from build123d import *

# Parameters (mm, degrees)
SKETCH1_W           = 45.974
SKETCH1_H           = 31.496
BOSS_EXTRUDE2_DEPTH = 17.78
BOSS_EXTRUDE6_DEPTH = 3.302


with BuildPart() as part:
    # Sketch1 → Boss-Extrude2 (new body)
    with BuildSketch(Plane(origin=(0, 0, 0), x_dir=(1, 0, 0), z_dir=(0, 1, 0))):
        with Locations((1.215537396, -0.182473566)):
            Rectangle(SKETCH1_W, SKETCH1_H)
    extrude(amount=BOSS_EXTRUDE2_DEPTH)

    # Sketch2 → Boss-Extrude6 (add)
    with BuildSketch(Plane.XZ):
        with BuildLine():
            Line((-21.771462604, 6.913473566), (-21.771462604, -6.548526434))
            Line((-21.771462604, -6.548526434), (-30.800796473, -4.778472942))
            ThreePointArc((-30.800796473, -4.778472942), (-31.824571926, -3.246797777), (-30.439504653, -2.032))
            Line((-30.439504653, -2.032), (-24.546579859, -2.032))
            ThreePointArc((-24.546579859, -2.032), (-22.514579859, 0), (-24.546579859, 2.032))
            Line((-24.546579859, 2.032), (-30.439504653, 2.032))
            ThreePointArc((-30.439504653, 2.032), (-31.827108275, 3.267243429), (-30.76084181, 4.78854089))
            Line((-30.76084181, 4.78854089), (-21.771462604, 6.913473566))
        make_face()
        with BuildLine():
            Line((32.870579445, 2.032), (26.977654651, 2.032))
            ThreePointArc((26.977654651, 2.032), (24.945654651, 0), (26.977654651, -2.032))
            Line((26.977654651, -2.032), (32.870579445, -2.032))
            ThreePointArc((32.870579445, -2.032), (34.255646718, -3.246797777), (33.231871264, -4.778472942))
            Line((33.231871264, -4.778472942), (24.202537396, -6.548526434))
            Line((24.202537396, -6.548526434), (24.202537396, 6.913473566))
            Line((24.202537396, 6.913473566), (33.191916602, 4.78854089))
            ThreePointArc((33.191916602, 4.78854089), (34.258183067, 3.267243429), (32.870579445, 2.032))
        make_face()
    extrude(amount=-BOSS_EXTRUDE6_DEPTH)


solid = part.part
Model file for the job. Use its own axes, mm. A direction names the side the tool comes from. Coordinates: 2 decimals unless noted, no trailing zeros. Write each loop counter-clockwise with the first axis right and the second up, starting at its lowest first coordinate (ties: lowest second). Pieces come first, ordered by that corner, then holes. Notation, with made-up numbers: (41.25, -23) - (63.25, -23) arc R23 ccw to (63.25, -11) - close; hole circle Ø1 at (64.25, 64). An arc over 180 degrees is marked (long way). Write each question's results on one line, items separated by ' | '. Start each with the question number.
1) Cut at D-D (z = 12.5). Write the cut outline in (x, y).
2) Mould opens along Z. For faces 4 (the face through (24.946, 1.628, 0.045)), 5 (the face through (-26.223, 1.628, -5.676)), 6 (the face through (1, 0, 0)) say: pulls with the +Z half, pulls with the -Z half, needs draft (parallel to the pull), parting line crosses it, or undercut.
3) Cut at C-C (y = 15.25). Write the cut outline in (x, z), then the cut area to 3 significant figures.
4) Probe line 1 along X through (y, z) = (14.75, 11.5); line 2 along Y through (x, z) = (29, 5); line 3 along X through (y, z) = (2.5, 2.5). List the from-to ranges inside material, lowest first. Write a range as from..to.
5) Cut at B-B (x = -26). Write the cut outline in (y, z).
6) Flat gauge pins, fed straight in: P1, Ø8, axis at y = 10.5, z = 4.5, coming from the +X side; P2, Ø2, axis at x = -24.5, y = 4, coming from the +Z side; P3, Ø3, axis at x = 28, z = -0.5, coming from the +Y side; P4, Ø5.5, axis at y = 7, z = 2, coming from the -X side. Where does each tip first touch, or does it go through?
7) Cut at A-A (z = 0). Write the cut outline in (x, y).
8) 3-axis set-ups, long thin cutter, end or side, ignore diameter. For faces 1 (the face through (-28, 2, -2.032)), 2 (the face through (28, 3.302, -3)), 3 (the face through (28.634, 1.628, 5.866)): which of +Z, -Z, +X, -X, +Y, -Y reach the whole face in a straight line?
Returned:
1) outline: (-21.77, 0) - (24.2, 0) - (24.2, 17.78) - (-21.77, 17.78) - close
2) face 4: undercut | face 5: pulls with the -Z half | face 6: needs draft
3) outline: (-21.77, -15.57) - (24.2, -15.57) - (24.2, 15.93) - (-21.77, 15.93) - close | area: 1,450 mm^2
4) line 1: -21.77..24.2 | line 2: 0..3.3 | line 3: -31.48..33.91
5) outline: (0, -5.72) - (3.3, -5.72) - (3.3, -2.03) - (0, -2.03) - close; (0, 2.03) - (3.3, 2.03) - (3.3, 5.91) - (0, 5.91) - close
6) P1: x = 24.2 | P2: z = 6.44 | P3: through | P4: x = -21.77
7) outline: (-22.51, 0) - (24.95, 0) - (24.95, 3.3) - (24.2, 3.3) - (24.2, 17.78) - (-21.77, 17.78) - (-21.77, 3.3) - (-22.51, 3.3) - close
8) face 1: -X, +Y, -Y | face 2: +Z, -Z, +X, +Y | face 3: +Z, +X, +Y, -Y
